Work out the finished part from the listing and answer in its coordinate system (mm). Face numbers are marked on the shaded views. A direction names the side the tool comes from. Round coordinates to 2 decimals unless told otherwise and drop trailing zeros. Order: outer loops, then holes, each group sorted by start corner. A loop starts at its lowest first (then second) coordinate and runs counter-clockwise, first axis right, second up. Notation, with made-up numbers: (1, 49.25) -> (47, 49.25) arc R33 ccw to (47, 86.25) -> close; hole circle Ø4 at (39, 16). An arc over 180 degrees is marked (long way). Use one line per item in the form item = value.
```python
from build123d import *

# Parameters (mm, degrees)
F0_R          = 3.6659795791
F1_DEPTH      = 2.286
F1_DEPTH_BACK = 2.286


with BuildPart() as f1:
    # F0 (on Top) → F1 (new body, two sides)
    with BuildSketch(Plane.XY) as f1_sk:
        with BuildLine():
            ThreePointArc((-10.7581636849, 38.5943156396), (-12.3120194853, 41.5236119371), (-12.2948130254, 44.8394751105))
            Line((-12.2948130254, 44.8394751105), (-32.1341768742, 37.5786978342))
            Line((-32.1341768742, 37.5786978342), (-36.8999519289, 27.4972548299))
            Line((-36.8999519289, 27.4972548299), (-31.4009838641, 27.4972548299))
            Line((-31.4009838641, 27.4972548299), (-28.6514998317, 31.071584724))
            Line((-28.6514998317, 31.071584724), (-23.3358272255, 28.9636466709))
            Line((-23.3358272255, 28.9636466709), (-20.0364456416, 33.5461209119))
            Line((-20.0364456416, 33.5461209119), (-12.8877867848, 33.5461209119))
            Line((-12.8877867848, 33.5461209119), (-10.7581636849, 38.5943156396))
        make_face()
        with BuildLine():
            Line((-5.712940873, 31.071584724), (-5.712940873, 36.3514380628))
            ThreePointArc((-5.712940873, 36.3514380628), (-8.4735917494, 36.9374208909), (-10.7581636849, 38.5943156396))
            Line((-10.7581636849, 38.5943156396), (-9.405106017, 33.179522777))
            Line((-9.405106017, 33.179522777), (-11.6046943605, 28.413749585))
            Line((-11.6046943605, 28.413749585), (-18.7533550799, 28.413749585))
            Line((-18.7533550799, 28.413749585), (-22.2360358477, 24.0145740621))
            Line((-22.2360358477, 24.0145740621), (-26.8185079933, 25.4809661359))
            Line((-26.8185079933, 25.4809661359), (-30.4844879449, 23.4646779076))
            Line((-30.4844879449, 23.4646779076), (-35.6168613673, 23.0980795399))
            Line((-35.6168613673, 23.0980795399), (-31.584283048, 17.9657079802))
            Line((-31.584283048, 17.9657079802), (-21.6861382962, 17.9657079802))
            Line((-21.6861382962, 17.9657079802), (-11.6046943605, 21.6316870005))
            Line((-11.6046943605, 21.6316870005), (-5.712940873, 31.071584724))
        make_face()
        with BuildLine():
            Line((-4.2532354575, 43.1473446608), (1.0829657251, 43.1473446608))
            ThreePointArc((1.0829657251, 43.1473446608), (-4.8601343001, 49.8895303182), (-12.2948130254, 44.8394751105))
            ThreePointArc((-12.2948130254, 44.8394751105), (-12.3120194853, 41.5236119371), (-10.7581636849, 38.5943156396))
            ThreePointArc((-10.7581636849, 38.5943156396), (-8.4735917494, 36.9374208909), (-5.712940873, 36.3514380628))
            Line((-5.712940873, 36.3514380628), (-5.712940873, 42.832795892))
            ThreePointArc((-5.712940873, 42.832795892), (-8.219106195, 48.883214202), (-2.168687885, 46.3770488799))
            ThreePointArc((-2.168687885, 46.3770488799), (-2.7350813629, 44.4550494051), (-4.2532354575, 43.1473446608))
        make_face()
        with BuildLine():
            ThreePointArc((-5.712940873, 36.3514380628), (-0.9075092332, 38.341913021), (1.0829657251, 43.1473446608))
            Line((1.0829657251, 43.1473446608), (-4.2532354575, 43.1473446608))
            ThreePointArc((-4.2532354575, 43.1473446608), (-4.9663350821, 42.9123253649), (-5.712940873, 42.832795892))
            Line((-5.712940873, 42.832795892), (-5.712940873, 36.3514380628))
        make_face()
        with BuildLine():
            Line((6.987059127, 35.5273446608), (6.987059127, 43.1473446608))
            Line((6.987059127, 43.1473446608), (1.0829657251, 43.1473446608))
            ThreePointArc((1.0829657251, 43.1473446608), (-0.9075092332, 38.341913021), (-5.712940873, 36.3514380628))
            Line((-5.712940873, 36.3514380628), (-5.712940873, 31.071584724))
            Line((-5.712940873, 31.071584724), (1.907059127, 31.071584724))
            Line((1.907059127, 31.071584724), (1.907059127, 24.3811724298))
            Line((1.907059127, 24.3811724298), (9.527059127, 24.3811724298))
            Line((9.527059127, 24.3811724298), (9.527059127, 16.3160171882))
            Line((9.527059127, 16.3160171882), (17.147059127, 16.3160171882))
            Line((17.147059127, 16.3160171882), (17.147059127, 12.6673446608))
            Line((17.147059127, 12.6673446608), (22.4627302145, 12.6673446608))
            Line((22.4627302145, 12.6673446608), (29.847059127, 12.6673446608))
            Line((29.847059127, 12.6673446608), (29.847059127, 20.2873446608))
            Line((29.847059127, 20.2873446608), (22.227059127, 20.2873446608))
            Line((22.227059127, 20.2873446608), (22.227059127, 27.9073446608))
            Line((22.227059127, 27.9073446608), (14.607059127, 27.9073446608))
            Line((14.607059127, 27.9073446608), (14.607059127, 35.5273446608))
            Line((14.607059127, 35.5273446608), (6.987059127, 35.5273446608))
        make_face()
        with BuildLine():
            Line((29.847059127, 12.6673446608), (22.4627302145, 12.6673446608))
            ThreePointArc((22.4627302145, 12.6673446608), (19.6683145281, 10.0001717736), (18.54095211, 6.3053613295))
            Line((18.54095211, 6.3053613295), (19.3654773553, 2.5420768229))
            ThreePointArc((19.3654773553, 2.5420768229), (31.449090173, 0.5210860144), (29.847059127, 12.6673446608))
        make_face()
        with Locations((26.1548946708, 2.2019967959)):
            Circle(F0_R, mode=Mode.SUBTRACT)
        with BuildLine():
            Line((22.4627302145, 12.6673446608), (17.147059127, 12.6673446608))
            Line((17.147059127, 12.6673446608), (18.54095211, 6.3053613295))
            ThreePointArc((18.54095211, 6.3053613295), (19.6683145281, 10.0001717736), (22.4627302145, 12.6673446608))
        make_face()
    extrude(amount=F1_DEPTH)
    extrude(f1_sk.sketch, amount=-F1_DEPTH_BACK)


solid = f1.part
```
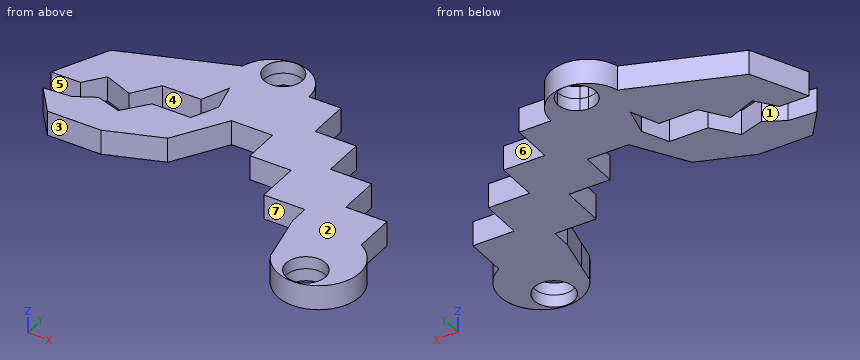
Item 1: Flat-ended cylindrical pins translate along their axes: P1, Ø4.5, axis at x = -5.71, y = 46.38, coming from the +Z side; P2, Ø1.1, axis at y = 15, z = 1, coming from the -X side; P3, Ø1.4, axis at x = -33, z = 0, coming from the -Y side; P4, Ø2.5, axis at y = 33, z = -1, coming from the +X side. Find the tip coordinate at first contact, or state that the pin passes through.
Findings:
P1 = through
P2 = 17.15
P3 = 18.88
P4 = 14.61
Item 2: The part is cut by section C-C, the plane x = 12. Give the vertices of the cut face in (y, z), and give its area (3 significant figures).
Findings:
outline = (16.32, -2.29) -> (35.53, -2.29) -> (35.53, 2.29) -> (16.32, 2.29) -> close
area = 87.8 mm^2
Item 3: Consider line 1 along Y through (x, z) = (13, 0.55); line 2 along X through (y, z) = (28, -2.05); line 3 along X through (y, z) = (22.5, 2.15). Determine where each line is inside the solid, lowest interval first.
Findings:
line_1 = 16.32 to 35.53
line_2 = -36.66 to -31.01, -19.08 to -7.63, 1.91 to 14.61
line_3 = -35.15 to -11.06, 9.53 to 22.23
Item 4: The part is cut by section B-B, the plane y = 15. Give the vertices of the cut face in (x, z).
Findings:
outline = (17.15, -2.29) -> (29.85, -2.29) -> (29.85, 2.29) -> (17.15, 2.29) -> close
Item 5: Determine the mould class of the marked faces 1, 2 and 3 for opening direction Y: released by +Y, released by -Y, zero draft, split by the parting line, or undercut.
Findings:
face_1 = undercut
face_2 = zero draft
face_3 = released by -Y
Item 6: For the marked faces 4, 5, 6 and 7, determine the directions among +Z, -Z, +X, -X, +Y, -Y from which every point of the face is accessible in a straight line to the end or side of a thin tool.
Findings:
face_4 = +Z, -Z
face_5 = +Z, -Z, -X
face_6 = +Z, -Z, +X, +Y
face_7 = +Z, -Z, -X, -Y
Item 7: The part is cut by section A-A, the plane x = -25. Give the vertices of the cut face in (y, z).
Findings:
outline = (17.97, -2.29) -> (24.9, -2.29) -> (24.9, 2.29) -> (17.97, 2.29) -> close; (29.62, -2.29) -> (40.19, -2.29) -> (40.19, 2.29) -> (29.62, 2.29) -> close
Item 8: The part is cut by section D-D, the plane z = 0.7. Give the number of separate pieces and of enclosed holes in the cut face, and give its area (3 significant figures).
Findings:
separate_pieces = 1
enclosed_holes = 2
area = 1,120 mm^2
